from build123d import *

# Parameters (mm, degrees)
BOSS_EXTRUDE1_DEPTH = 50
CUT_EXTRUDE1_DEPTH  = 7.5
LPATTERN1_COUNT     = 4
LPATTERN1_PITCH     = 25


with BuildPart() as part:
    # Sketch1 → Boss-Extrude1 (new, symmetric)
    with BuildSketch(Plane.XY):
        with BuildLine():
            Line((7.5, 17.5), (6.5, 17.5))
            Line((6.5, 17.5), (6.5, 14))
            ThreePointArc((6.5, 14), (6.353553391, 13.646446609), (6, 13.5))
            Line((6, 13.5), (1, 13.5))
            ThreePointArc((1, 13.5), (0.292893219, 13.207106781), (0, 12.5))
            Line((0, 12.5), (0, -12.5))
            ThreePointArc((0, -12.5), (0.292893219, -13.207106781), (1, -13.5))
            Line((1, -13.5), (6, -13.5))
            ThreePointArc((6, -13.5), (6.353553391, -13.646446609), (6.5, -14))
            Line((6.5, -14), (6.5, -17.5))
            Line((6.5, -17.5), (7.5, -17.5))
            Line((7.5, -17.5), (7.5, -13.5))
            ThreePointArc((7.5, -13.5), (7.207106781, -12.792893219), (6.5, -12.5))
            Line((6.5, -12.5), (1.5, -12.5))
            ThreePointArc((1.5, -12.5), (1.146446609, -12.353553391), (1, -12))
            Line((1, -12), (1, 12))
            ThreePointArc((1, 12), (1.146446609, 12.353553391), (1.5, 12.5))
            Line((1.5, 12.5), (6.5, 12.5))
            ThreePointArc((6.5, 12.5), (7.207106781, 12.792893219), (7.5, 13.5))
            Line((7.5, 13.5), (7.5, 17.5))
        make_face()
    extrude(amount=BOSS_EXTRUDE1_DEPTH, both=True)

    # Sketch2 → Cut-Extrude1 (cut)
    with BuildSketch(Plane(origin=(0, 0, 0), x_dir=(0, 0, -1), z_dir=(1, 0, 0))):
        with BuildLine():
            Line((-43.35, 3.15), (-31.65, 3.15))
            ThreePointArc((-31.65, 3.15), (-28.5, 0), (-31.65, -3.15))
            Line((-31.65, -3.15), (-43.35, -3.15))
            ThreePointArc((-43.35, -3.15), (-46.5, 0), (-43.35, 3.15))
        make_face()
    cut_extrude1 = extrude(amount=CUT_EXTRUDE1_DEPTH, mode=Mode.SUBTRACT)

    # LPattern1: Cut-Extrude1 ×4
    with Locations(*[(0, 0, -i * LPATTERN1_PITCH) for i in range(1, LPATTERN1_COUNT)]):
        add(cut_extrude1, mode=Mode.SUBTRACT)


solid = part.part
Geometry: final body of the model. Coordinates: model frame, mm. A direction names the side the tool comes from. Round coordinates to 2 decimals unless told otherwise and drop trailing zeros. Order: outer loops, then holes, each group sorted by start corner. A loop starts at its lowest first (then second) coordinate and runs counter-clockwise, first axis right, second up.
Q1. Section C-C, the plane y = 0. Output: boundary loops of the cut face in (x, z).
Result sheet:
outline: (0, -50) - (1, -50) - (1, -46.5) - (0, -46.5) - close; (0, -28.5) - (1, -28.5) - (1, -21.5) - (0, -21.5) - close; (0, -3.5) - (1, -3.5) - (1, 3.5) - (0, 3.5) - close; (0, 21.5) - (1, 21.5) - (1, 28.5) - (0, 28.5) - close; (0, 46.5) - (1, 46.5) - (1, 50) - (0, 50) - close
Q2. Section A-A, the plane x = 3.25. Output: boundary loops of the cut face in (y, z).
Result sheet:
outline: (-13.5, -50) - (-12.5, -50) - (-12.5, 50) - (-13.5, 50) - close; (12.5, -50) - (13.5, -50) - (13.5, 50) - (12.5, 50) - close
Q3. Section B-B, the plane z = 33. Output: boundary loops of the cut face in (x, y), and give its area (3 significant figures).
Result sheet:
outline: (0, -12.5) arc R1 ccw to (1, -13.5) - (6, -13.5) arc R0.5 cw to (6.5, -14) - (6.5, -17.5) - (7.5, -17.5) - (7.5, -13.5) arc R1 ccw to (6.5, -12.5) - (1.5, -12.5) arc R0.5 cw to (1, -12) - (1, -3.15) - (0, -3.15) - close; (0, 3.15) - (1, 3.15) - (1, 12) arc R0.5 cw to (1.5, 12.5) - (6.5, 12.5) arc R1 ccw to (7.5, 13.5) - (7.5, 17.5) - (6.5, 17.5) - (6.5, 14) arc R0.5 cw to (6, 13.5) - (1, 13.5) arc R1 ccw to (0, 12.5) - close
area: 41.1 mm2
Q4. Section D-D, the plane y = 15. Output: boundary loops of the cut face in (x, z), and give its area (3 significant figures).
Result sheet:
outline: (6.5, -50) - (7.5, -50) - (7.5, 50) - (6.5, 50) - close
area: 100 mm2
Q5. Access query for faces 1 (the face through (4, -12.5, 1)), 2 (the face through (3, -13.5, 1)), 3 (the face through (0.5, 0.1, 3.5)). Directions: +Z, -Z, +X, -X, +Y, -Y. A direction counts if a zero-diameter tool reaches every point of the face in a straight line with its end or side. Return the directions, or none.
Result sheet:
face 1: +Z, -Z, +X
face 2: +Z, -Z, -X, -Y
face 3: +X, -X
Q6. Material intervals for probe 1 along Y at (x, z) = (5.75, 21); probe 2 along X at (y, z) = (-15, 29.5); probe 3 along X at (y, z) = (-7, -21), sorted ascending.
Result sheet:
probe 1: y = -13.5 to -12.5, 12.5 to 13.5
probe 2: x = 6.5 to 7.5
probe 3: x = 0 to 1
Q7. Pin query (flat end, axial travel): pin 1 (4 mm diameter, centred on x = 3.5, z = 14.5, fed in from -Y); pin 2 (1.8 mm diameter, centred on y = 16, z = -3, fed in from -X); pin 3 (1.1 mm diameter, centred on x = 0.5, z = -37, fed in from +Y). Return the tip coordinate at first contact, or that it passes through.
Result sheet:
pin 1: stops at y = -13.5
pin 2: stops at x = 6.5
pin 3: stops at y = 13.5
Q8. Mould query, pull axis Z, two halves, no side actions, for faces 4 (the face through (4, 12.5, 1)), 5 (the face through (0.5, -0.1, -28.5)), 6 (the face through (0.7, -1.2, -50)). Classes: released by +Z, released by -Z, zero draft, split by the parting line, or undercut.
Result sheet:
face 4: zero draft
face 5: undercut
face 6: released by -Z
